Job drawing, mm, ordinate dimensions from the low corner. One solid piece. Coordinates: 2 decimals unless noted, no trailing zeros. Write each loop counter-clockwise with the first axis right and the second up, starting at its lowest first coordinate (ties: lowest second). Pieces come first, ordered by that corner, then holes. Notation, with made-up numbers: (-1, 33.5) - (32, 33.5) arc R23 ccw to (32, 69.5) - close; hole circle Ø6 at (71, -36.5). An arc over 180 degrees is marked (long way). Use one line per item in the form item = value. Start each with the question number.
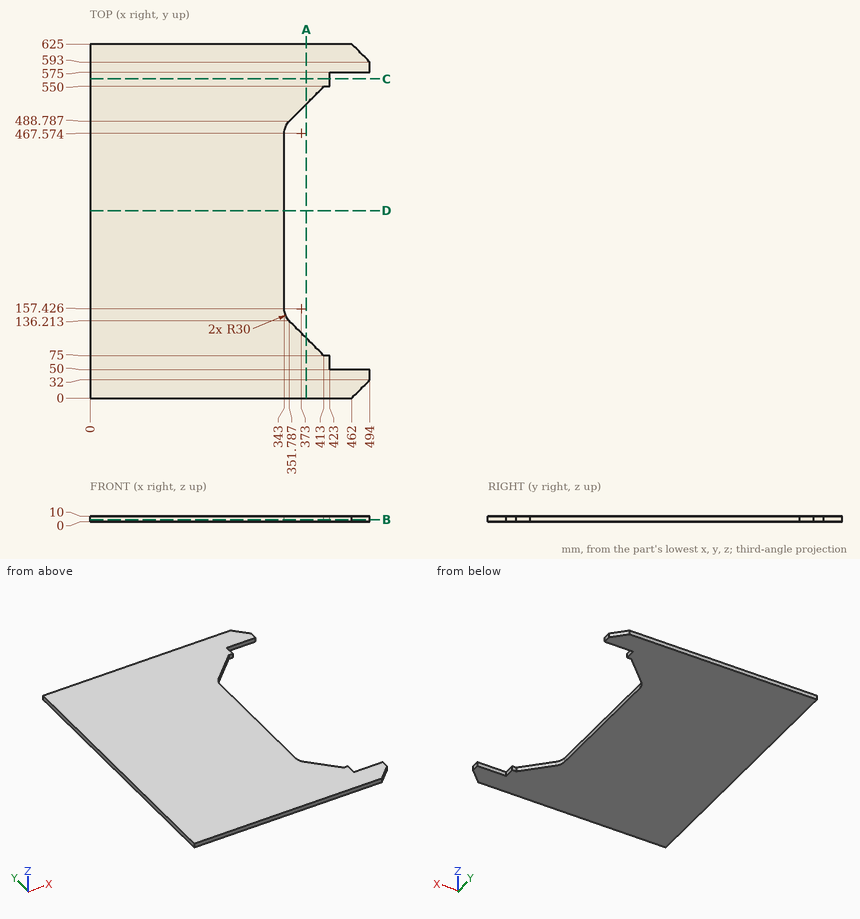
Q1. Slice it at C-C (y = 563.5). List the corners of the cut face in (x, z), plus the area to 3 significant figures.
Q2. Pin check, flat tips, straight feed: P1, Ø5, axis at y = 564, z = 2.5, coming from the +X side; P2, Ø3, axis at y = 381.5, z = 7, coming from the +X side. Stop position of each tip, or through.
Q3. Slice it at D-D (y = 331). List the corners of the cut face in (x, z).
Q4. Slice it at B-B (z = 3.75). List the corners of the cut face in (x, y).
Q5. Slice it at A-A (x = 382). List the corners of the cut face in (y, z), plus the area to 3 significant figures.
Q6. Drill centre lines: probe 1 along Y at (x, z) = (425.5, 7.5); probe 2 along X at (y, z) = (276.5, 3.25); probe 3 along X at (y, z) = (68.5, 8.5). Where is each one in solid material? Low to high.
Solution:
q1.outline = (0, 0) - (423, 0) - (423, 10) - (0, 10) - close
q1.area = 4,230 mm2
q2.P1 = 423
q2.P2 = 343
q3.outline = (0, 0) - (343, 0) - (343, 10) - (0, 10) - close
q4.outline = (0, 0) - (462, 0) - (494, 32) - (494, 50) - (423, 50) - (423, 75) - (413, 75) - (351.79, 136.21) arc R30 cw to (343, 157.43) - (343, 467.57) arc R30 cw to (351.79, 488.79) - (413, 550) - (423, 550) - (423, 575) - (494, 575) - (494, 593) - (462, 625) - (0, 625) - close
q5.outline = (0, 0) - (106, 0) - (106, 10) - (0, 10) - close; (519, 0) - (625, 0) - (625, 10) - (519, 10) - close
q5.area = 2,120 mm2
q6.probe_1 = 0 to 50, 575 to 625
q6.probe_2 = 0 to 343
q6.probe_3 = 0 to 423
